Source: three-view drawing plus pictorial views. Frame: mm from the lowest corner of the part. Give positions to 0.01 mm unless a question says otherwise; leave off trailing zeros. Loops run counter-clockwise (first coordinate to the right, second up) from the corner with the lowest first, then second, coordinate; pieces in that order, holes last. Notation, with made-up numbers: (-6.5, 84.5) -> (8.5, 84.5) arc R9 ccw to (8.5, 98.5) -> close; hole circle Ø2 at (-19, -39.5). An arc over 180 degrees is marked (long way). Answer as a JSON object with one key per item and string values. Group by question number.
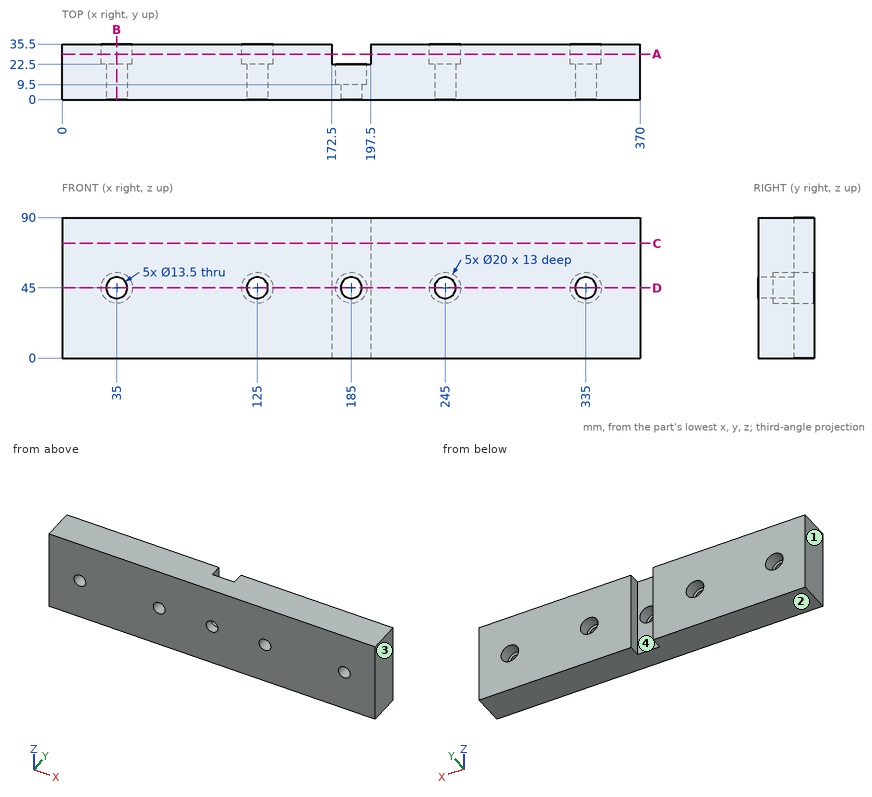
Q1. Section A-A on y = 29. Return the cut outline in (x, z).
Q2. Section B-B on x = 35. Return the cut outline in (y, z).
Q3. Ray query, probe 1 along X at (y, z) = (6.25, 45); probe 2 along X at (y, z) = (29, 45); probe 3 along Z at (x, y) = (334.5, 25). Return the intervals inside material, ascending.
Q4. Pull-direction query (X, two-part tool) for the marked faces 1, 2, 3 and 4; classes: +X half, -X half, draft (parallel to the pull), parting line (faces both ways), or undercut.
Q5. Section C-C on z = 73.5. Return the cut outline in (x, y).
Q6. Section D-D on z = 45. State how many separate pieces and enclosed holes the cut face has, then the cut area to 3 significant figures.
Q7. Pin query (flat end, axial travel): pin 1 Ø1 at (x, z) = (187.5, 16.5) entering from +Y; pin 2 Ø10 at (x, z) = (334, 45.5) entering from +Y. Return the tip coordinate at first contact, or that it passes through.
Numbers:
{
 "1": {"outline": "(0, 0) -> (172.5, 0) -> (172.5, 90) -> (0, 90) -> close; (197.5, 0) -> (370, 0) -> (370, 90) -> (197.5, 90) -> close; hole circle Ø20 at (35, 45); hole circle Ø20 at (125, 45); hole circle Ø20 at (245, 45); hole circle Ø20 at (335, 45)"},
 "2": {"outline": "(0, 0) -> (35.5, 0) -> (35.5, 35) -> (22.5, 35) -> (22.5, 38.25) -> (0, 38.25) -> close; (0, 51.75) -> (22.5, 51.75) -> (22.5, 55) -> (35.5, 55) -> (35.5, 90) -> (0, 90) -> close"},
 "3": {"probe 1": "x = 0 to 28.25, 41.75 to 118.25, 131.75 to 178.25, 191.75 to 238.25, 251.75 to 328.25, 341.75 to 370", "probe 2": "x = 0 to 25, 45 to 115, 135 to 172.5, 197.5 to 235, 255 to 325, 345 to 370", "probe 3": "z = 0 to 35.01, 54.99 to 90"},
 "4": {"face 1": "-X half", "face 2": "draft", "face 3": "+X half", "face 4": "undercut"},
 "5": {"outline": "(0, 0) -> (370, 0) -> (370, 35.5) -> (197.5, 35.5) -> (197.5, 22.5) -> (172.5, 22.5) -> (172.5, 35.5) -> (0, 35.5) -> close"},
 "6": {"separate pieces": "6", "enclosed holes": "0", "area": "10,200 mm²"},
 "7": {"pin 1": "stops at y = 22.5", "pin 2": "passes through"}
}
